Build history of the part. All positions in model axes, mm. A direction names the side the tool comes from. Round coordinates to 2 decimals unless told otherwise and drop trailing zeros. Order: outer loops, then holes, each group sorted by start corner. A loop starts at its lowest first (then second) coordinate and runs counter-clockwise, first axis right, second up. Notation, with made-up numbers: (6.25, 55.25) -> (46.25, 55.25) arc R11 cw to (46.25, 73.25) -> close; hole circle Ø5 at (16, 53.5). An arc over 180 degrees is marked (long way). Answer as a JSON object with one key per item and string values.
from build123d import *

# Parameters (mm, degrees)
SKETCH1_R           = 3.4925
SKETCH1_R_2         = 0.9525
BOSS_EXTRUDE1_DEPTH = 2.54


with BuildPart() as part:
    # Sketch1 → Boss-Extrude1 (new body)
    with BuildSketch(Plane(origin=(0, 0, 0), x_dir=(1, 0, 0), z_dir=(0, 1, 0))):
        with BuildLine():
            Line((-20.195257301, 13.738549126), (-20.195257301, -13.738549126))
            ThreePointArc((-20.195257301, -13.738549126), (-22.109488558, -22.158548823), (-13.716417781, -20.1295))
            Line((-13.716417781, -20.1295), (13.716417781, -20.1295))
            ThreePointArc((13.716417781, -20.1295), (22.109488558, -22.158548823), (20.195257301, -13.738549126))
            Line((20.195257301, -13.738549126), (20.195257301, 13.738549126))
            ThreePointArc((20.195257301, 13.738549126), (22.109488558, 22.158548823), (13.716417781, 20.1295))
            Line((13.716417781, 20.1295), (-13.716417781, 20.1295))
            ThreePointArc((-13.716417781, 20.1295), (-22.109488558, 22.158548823), (-20.195257301, 13.738549126))
        make_face()
        with Locations(Location((18.542, -18.542, 0), (0, 0, 270))):
            Circle(SKETCH1_R, mode=Mode.SUBTRACT)
        with Locations(Location((-18.542, -18.542, 0), (0, 0, 270))):
            Circle(SKETCH1_R, mode=Mode.SUBTRACT)
        with Locations(Location((-18.542, 18.542, 0), (0, 0, 270))):
            Circle(SKETCH1_R, mode=Mode.SUBTRACT)
        with Locations(Location((18.542, 18.542, 0), (0, 0, 270))):
            Circle(SKETCH1_R, mode=Mode.SUBTRACT)
        with Locations(Location((-13.969691774, 0, 0), (0, 0, 270))):
            Circle(SKETCH1_R_2, mode=Mode.SUBTRACT)
        with Locations(Location((13.969691774, 0, 0), (0, 0, 270))):
            Circle(SKETCH1_R_2, mode=Mode.SUBTRACT)
        with BuildLine():
            Line((-17.020257301, 13.695279546), (-17.020257301, 1.27))
            Line((-17.020257301, 1.27), (-13.969691774, 1.27))
            ThreePointArc((-13.969691774, 1.27), (-12.699691774, 0), (-13.969691774, -1.27))
            Line((-13.969691774, -1.27), (-17.020257301, -1.27))
            Line((-17.020257301, -1.27), (-17.020257301, -13.695279546))
            ThreePointArc((-17.020257301, -13.695279546), (-14.974400962, -14.925560161), (-13.716417781, -16.9545))
            Line((-13.716417781, -16.9545), (13.716417781, -16.9545))
            ThreePointArc((13.716417781, -16.9545), (14.974400962, -14.925560161), (17.020257301, -13.695279546))
            Line((17.020257301, -13.695279546), (17.020257301, -1.27))
            Line((17.020257301, -1.27), (13.969691774, -1.27))
            ThreePointArc((13.969691774, -1.27), (12.699691774, 0), (13.969691774, 1.27))
            Line((13.969691774, 1.27), (17.020257301, 1.27))
            Line((17.020257301, 1.27), (17.020257301, 13.695279546))
            ThreePointArc((17.020257301, 13.695279546), (14.974400962, 14.925560161), (13.716417781, 16.9545))
            Line((13.716417781, 16.9545), (-13.716417781, 16.9545))
            ThreePointArc((-13.716417781, 16.9545), (-14.974400962, 14.925560161), (-17.020257301, 13.695279546))
        make_face(mode=Mode.SUBTRACT)
    extrude(amount=BOSS_EXTRUDE1_DEPTH)


solid = part.part
1) Cut at A-A, the plane x = 11. Give the cut face in (y, z).
Checked values:
{"outline": "(0, -20.13) -> (2.54, -20.13) -> (2.54, -16.95) -> (0, -16.95) -> close; (0, 16.95) -> (2.54, 16.95) -> (2.54, 20.13) -> (0, 20.13) -> close"}
2) Cut at C-C, the plane y = 1.1. Count the separate pieces of the cut face and the enclosed holes in it, plus the area to 3 significant figures.
Checked values:
{"separate pieces": "1", "enclosed holes": "7", "area": "530 mm²"}
3) Flat gauge pins, fed straight in: pin 1 Ø1.5 at (y, z) = (0.5, 13.5) entering from -X; pin 2 Ø0.8 at (x, y) = (1.5, 1) entering from -Z; pin 3 Ø0.8 at (y, z) = (0.5, 3) entering from +X; pin 4 Ø1.5 at (x, z) = (-13.97, 0) entering from +Y. Where does each tip first touch, or does it go through?
Checked values:
{"pin 1": "stops at x = -21.26", "pin 2": "stops at z = -20.13", "pin 3": "stops at x = 20.2", "pin 4": "passes through"}
4) Pull direction Z, two halves, no side cores. Call faces 1 (the face through (22.005, 1.252, 22.259)), 2 (the face through (16, 2.54, 0)), 3 (the face through (0, 1, -20.13)), 4 (the face through (16.42, 1.25, 15.77)): pulls with the +Z half, pulls with the -Z half, needs draft (parallel to the pull), parting line crosses it, or undercut.
Checked values:
{"face 1": "undercut", "face 2": "needs draft", "face 3": "pulls with the -Z half", "face 4": "undercut"}
5) Which spindle directions (+Z, -Z, +X, -X, +Y, -Y) get a long thin tool onto all of the face, cutting with end or side? Do faces 5 (the face through (-20.195, 1, 0)), 6 (the face through (12.7, 1.3, 0)), 7 (the face through (16, 0, 0)). Say none if no direction does.
Checked values:
{"face 5": "-X, +Y, -Y", "face 6": "+Y, -Y", "face 7": "+Z, -Z, +X, -X, -Y"}
6) Probe L1, parallel to Z at x = -3, y = 0.65; L2, parallel to X at y = 1.95, z = -5; L3, parallel to Z at x = 16, y = 1.8. List the from-to ranges inside material, lowest first. Write a range as from..to.
Checked values:
{"L1": "z = -20.13..-16.95, 16.95..20.13", "L2": "x = -20.2..-17.02, 17.02..20.2", "L3": "z = -22.94..-20.94, -16.15..-14.14, -1.27..1.27, 14.14..16.15, 20.94..22.94"}
7) Cut at D-D, the plane x = -18. Give the cut face in (y, z).
Checked values:
{"outline": "(0, -23.59) -> (2.54, -23.59) -> (2.54, -21.99) -> (0, -21.99) -> close; (0, -15.09) -> (2.54, -15.09) -> (2.54, 15.09) -> (0, 15.09) -> close; (0, 21.99) -> (2.54, 21.99) -> (2.54, 23.59) -> (0, 23.59) -> close"}
8) Cut at B-B, the plane z = -4. Give the cut face in (x, y), plus the area to 3 significant figures.
Checked values:
{"outline": "(-20.2, 0) -> (-17.02, 0) -> (-17.02, 2.54) -> (-20.2, 2.54) -> close; (17.02, 0) -> (20.2, 0) -> (20.2, 2.54) -> (17.02, 2.54) -> close", "area": "16.1 mm²"}
